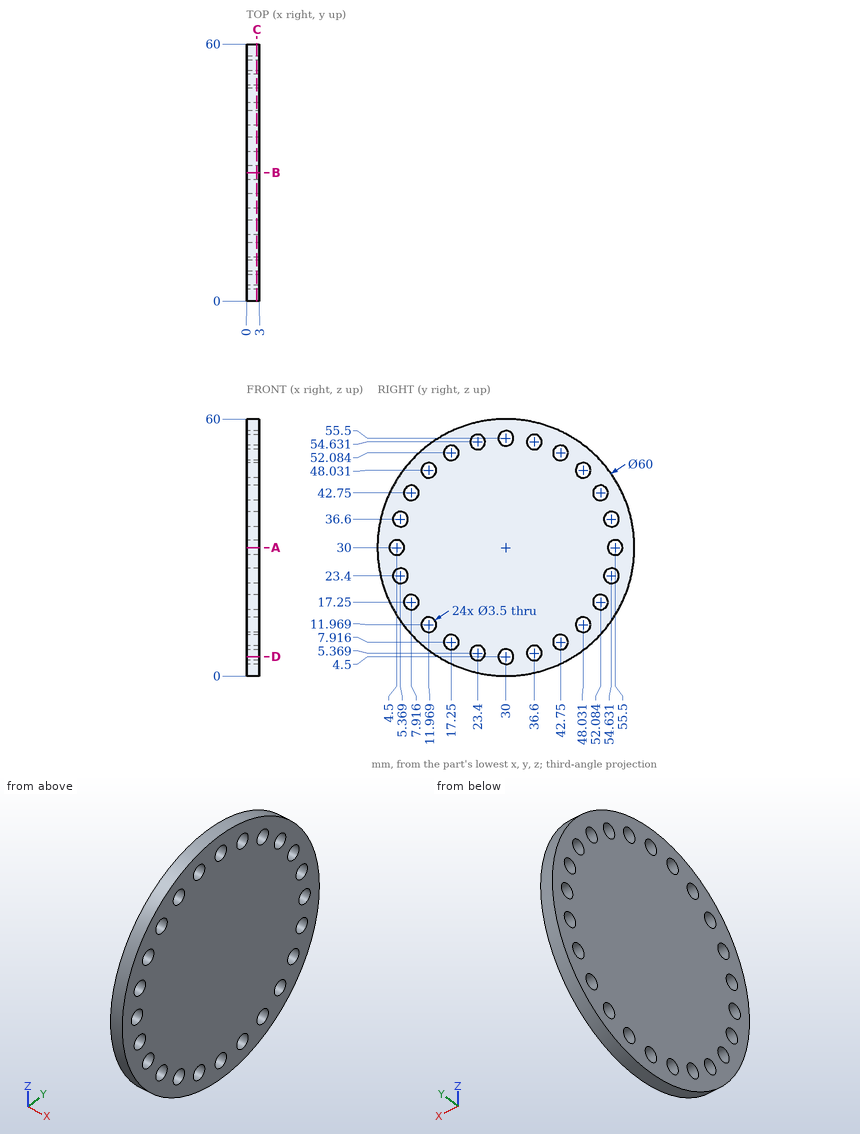
Print and shaded views of the part. All mm, measured from the part's lowest x, y and z. Give positions to 0.01 mm unless a question says otherwise; leave off trailing zeros. Loops run counter-clockwise (first coordinate to the right, second up) from the corner with the lowest first, then second, coordinate; pieces in that order, holes last. Notation, with made-up numbers: (-20, 86) - (-4, 86) arc R10 cw to (-4, 103) - close; hole circle Ø1 at (81.25, 29). An arc over 180 degrees is marked (long way). One line per item, written item: value. Start each with the question number.
1. Slice it at D-D (z = 4.5). List the corners of the cut face in (x, y).
2. Pin check, flat tips, straight feed: pin 1 (1.5 mm diameter, centred on x = 2, z = 32.5, fed in from +Y); pin 2 (1 mm diameter, centred on x = 2, z = 45, fed in from +Y). Stop position of each tip, or through.
3. Slice it at A-A (z = 30). List the corners of the cut face in (x, y), plus the area to 3 significant figures.
4. Probe L1, parallel to Y at x = 1.2, z = 8.5; L2, parallel to Y at x = 1.6, z = 42 (1 decimal); L3, parallel to Z at x = 1.95, y = 6 (1 decimal). List the from-to ranges inside material, lowest first. Write a range as from..to.
5. Slice it at C-C (x = 2.4). Give the number of separate pieces and of enclosed holes in the cut face, plus the area to 3 significant figures.
Solution:
1. outline: (0, 14.2) - (3, 14.2) - (3, 21.88) - (0, 21.88) - close; (0, 24.92) - (3, 24.92) - (3, 28.25) - (0, 28.25) - close; (0, 31.75) - (3, 31.75) - (3, 35.08) - (0, 35.08) - close; (0, 38.12) - (3, 38.12) - (3, 45.8) - (0, 45.8) - close
2. pin 1: stops at y = 59.95
2. pin 2: stops at y = 56.26
3. outline: (0, 0) - (3, 0) - (3, 2.75) - (0, 2.75) - close; (0, 6.25) - (3, 6.25) - (3, 53.75) - (0, 53.75) - close; (0, 57.25) - (3, 57.25) - (3, 60) - (0, 60) - close
3. area: 159 mm^2
4. L1: y = 9.08..15.6, 18.9..41.1, 44.4..50.92
4. L2: y = 2.5..6.3, 9.5..50.5, 53.7..57.5
4. L3: z = 12..21.8, 25..29.1, 30.9..35, 38.2..48
5. separate pieces: 1
5. enclosed holes: 24
5. area: 2,600 mm^2
